The figure shows three views and two pictorial views of one solid part (mm, origin at its lowest corner). Answer the questions. Give positions to 0.01 mm unless a question says otherwise; leave off trailing zeros. Order: outer loops, then holes, each group sorted by start corner. A loop starts at its lowest first (then second) coordinate and runs counter-clockwise, first axis right, second up. Notation, with made-up numbers: M 38,1.25 L 75,1.25 A26 cw 75,39.25 Z; hole C 71.5,86.5 d10. An arc over 180 degrees is marked long. Write item = value, one per line. Start each with the question number.
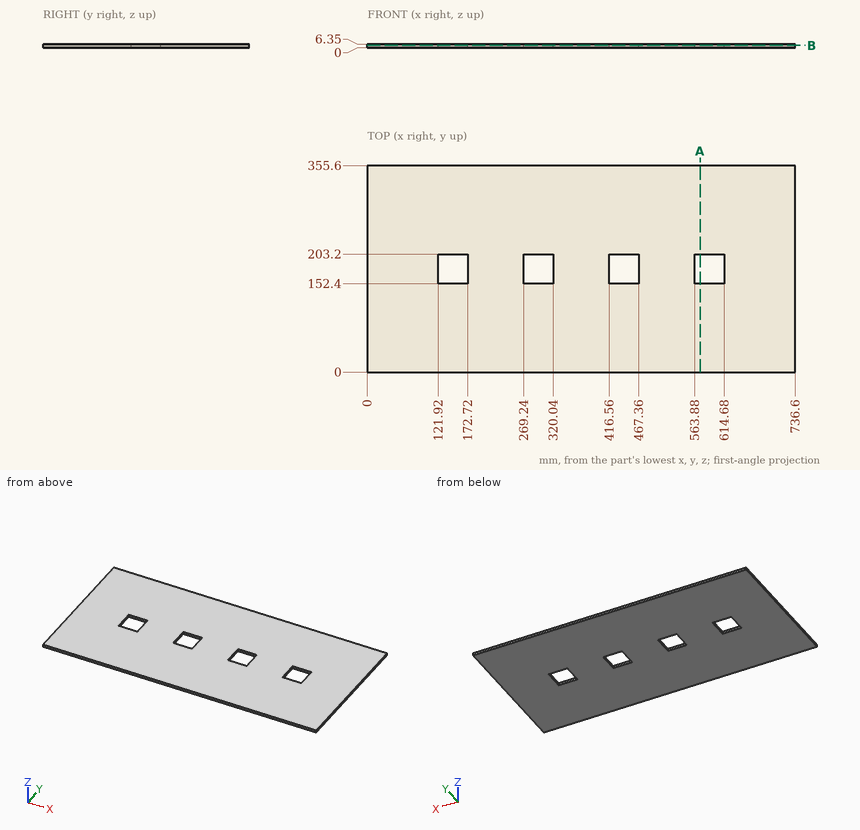
1) Find section A-A on x = 573. Determine the outline of the cut face in (y, z).
2) Find section B-B on z = 4. Determine the outline of the cut face in (x, y), plus the area to 3 significant figures.
3) Find the intervals of material crossed by probe 1 along X at (y, z) = (172, 1.25); probe 2 along Y at (x, z) = (600, 0.5), in increasing order. Write a range as [from, to].
Numbers:
q1.outline = M 0,0 L 152.4,0 L 152.4,6.35 L 0,6.35 Z; M 203.2,0 L 355.6,0 L 355.6,6.35 L 203.2,6.35 Z
q2.outline = M 0,0 L 736.6,0 L 736.6,355.6 L 0,355.6 Z; hole M 121.92,152.4 L 172.72,152.4 L 172.72,203.2 L 121.92,203.2 Z; hole M 269.24,152.4 L 320.04,152.4 L 320.04,203.2 L 269.24,203.2 Z; hole M 416.56,152.4 L 467.36,152.4 L 467.36,203.2 L 416.56,203.2 Z; hole M 563.88,152.4 L 614.68,152.4 L 614.68,203.2 L 563.88,203.2 Z
q2.area = 252,000 mm2
q3.probe_1 = [0, 121.92], [172.72, 269.24], [320.04, 416.56], [467.36, 563.88], [614.68, 736.6]
q3.probe_2 = [0, 152.4], [203.2, 355.6]
